```python
from build123d import *

# Parameters (mm, degrees)
SKETCH2_W           = 170
SKETCH2_H           = 75
BOSS_EXTRUDE2_DEPTH = 5
EXTRUDE_THIN1_START = 5
SKETCH2_3_W         = 170
SKETCH2_3_H         = 75
SKETCH2_3_W_2       = 164
SKETCH2_3_H_2       = 69
EXTRUDE_THIN1_DEPTH = 65
SKETCH2_6_R         = 2.2
CUT_EXTRUDE1_DEPTH  = 6


with BuildPart() as part:
    # Sketch2 → Boss-Extrude2 (new body)
    with BuildSketch(Plane(origin=(0, 0, 0), x_dir=(1, 0, 0), z_dir=(0, 1, 0))):
        Rectangle(SKETCH2_W, SKETCH2_H)
    extrude(amount=BOSS_EXTRUDE2_DEPTH)

    # Sketch2<3> → Extrude-Thin1 (add)
    with BuildSketch(Plane(origin=(0, 0, 0), x_dir=(1, 0, 0), z_dir=(0, 1, 0)).offset(EXTRUDE_THIN1_START)):
        Rectangle(SKETCH2_3_W, SKETCH2_3_H)
        Rectangle(SKETCH2_3_W_2, SKETCH2_3_H_2, mode=Mode.SUBTRACT)
    extrude(amount=EXTRUDE_THIN1_DEPTH)

    # Sketch2<6> → Cut-Extrude1 (cut)
    with BuildSketch(Plane(origin=(0, 0, 0), x_dir=(1, 0, 0), z_dir=(0, 1, 0))):
        with Locations(Location((-67.65, 14.9, 0), (0, 0, 270))):
            Circle(SKETCH2_6_R)
        with Locations(Location((67.65, 14.9, 0), (0, 0, 90))):
            Circle(SKETCH2_6_R)
        with Locations(Location((67.65, -27.9, 0), (0, 0, 270))):
            Circle(SKETCH2_6_R)
        with Locations(Location((-67.65, -27.9, 0), (0, 0, 90))):
            Circle(SKETCH2_6_R)
    extrude(amount=CUT_EXTRUDE1_DEPTH, mode=Mode.SUBTRACT)


solid = part.part
```
For this review, take the finished solid that the model builds, in its own axes (mm). A direction names the side the tool comes from. Round coordinates to 2 decimals unless told otherwise and drop trailing zeros. Write each loop counter-clockwise with the first axis right and the second up, starting at its lowest first coordinate (ties: lowest second). Pieces come first, ordered by that corner, then holes. Notation, with made-up numbers: (77, 9.5) - (135, 9.5) arc R25 cw to (135, 21.5) - close; hole circle Ø10 at (28.25, 72). An arc over 180 degrees is marked (long way). Answer as CSV lines item,"result". Start each with the question number.
(1) Add section B-B, the plane x = -67.65. State the section outline as (y, z) points, plus the area to 3 significant figures.
(2) Machinability: for faces 5 (the flat face through (-26, 70, 36)), 6 (the flat face through (-1, 37, -34.5)), which of the approach directions +Z, -Z, +X, -X, +Y, -Y give a long, thin tool a straight path to every point of the face, cutting with its end or side? Answer none if there is none.
(3) Add section C-C, the plane y = 54.5. State the section outline as (x, z) points.
(4) For line 1 (Z direction, x = -67.65, y = 2.75); line 2 (X direction, y = 1.2, z = -14.9); line 3 (Z direction, x = -58.5, y = 47.5), list the stretches that pass through material, from the lowest coordinate up.
(5) For pin 1 (5.5 mm diameter, centred on x = 67.65, z = -14.9, fed in from +Y); pin 2 (3.5 mm diameter, centred on x = -67.65, z = -14.9, fed in from +Y), all flat-tipped, find the tip position at first contact; note any pin that passes through.
(6) Add section A-A, the plane z = 27.9. State the section outline as (x, y) points, plus the area to 3 significant figures.
(7) Add section D-D, the plane z = 19. State the section outline as (x, y) points.
(8) Mouldability with a two-part tool opening along Z and no side actions: class faces 1 (the flat face through (-1, 35, -37.5)), 2 (the flat face through (82, 37, 0)), 3 (the flat face through (-1, 35, 37.5)), 4 (the flat face through (-85, 35, 1)) as +Z half, -Z half, draft (parallel to the pull), parting line (faces both ways), or undercut.
From the geometry:
1,outline,"(0, -37.5) - (70, -37.5) - (70, -34.5) - (5, -34.5) - (5, -17.1) - (0, -17.1) - close; (0, -12.7) - (5, -12.7) - (5, 25.7) - (0, 25.7) - close; (0, 30.1) - (5, 30.1) - (5, 34.5) - (70, 34.5) - (70, 37.5) - (0, 37.5) - close"
1,area,"721 mm²"
2,face 5,"+Z, -Z, +X, -X, +Y"
2,face 6,"+Y"
3,outline,"(-85, -37.5) - (85, -37.5) - (85, 37.5) - (-85, 37.5) - close; hole (-82, -34.5) - (82, -34.5) - (82, 34.5) - (-82, 34.5) - close"
4,line 1,"z = -37.5 to -17.1, -12.7 to 25.7, 30.1 to 37.5"
4,line 2,"x = -85 to -69.85, -65.45 to 65.45, 69.85 to 85"
4,line 3,"z = -37.5 to -34.5, 34.5 to 37.5"
5,pin 1,"stops at y = 5"
5,pin 2,"passes through"
6,outline,"(-85, 0) - (-69.85, 0) - (-69.85, 5) - (-82, 5) - (-82, 70) - (-85, 70) - close; (-65.45, 0) - (65.45, 0) - (65.45, 5) - (-65.45, 5) - close; (69.85, 0) - (85, 0) - (85, 70) - (82, 70) - (82, 5) - (69.85, 5) - close"
6,area,"1,200 mm²"
7,outline,"(-85, 0) - (85, 0) - (85, 70) - (82, 70) - (82, 5) - (-82, 5) - (-82, 70) - (-85, 70) - close"
8,face 1,"-Z half"
8,face 2,"undercut"
8,face 3,"+Z half"
8,face 4,"draft"
